Build history of the part. All positions in model axes, mm. A direction names the side the tool comes from. Round coordinates to 2 decimals unless told otherwise and drop trailing zeros. Write each loop counter-clockwise with the first axis right and the second up, starting at its lowest first coordinate (ties: lowest second). Pieces come first, ordered by that corner, then holes. Notation, with made-up numbers: (9, 54.25) -> (47, 54.25) arc R13 cw to (47, 69.25) -> close; hole circle Ø7 at (78.5, 38.5). An arc over 180 degrees is marked (long way). Return JSON: item names as keys, results as strings.
from build123d import *

# Parameters (mm, degrees)
ESQUISSE1_R       = 12
EXTRUSION1_DEPTH  = 12
ESQUISSE2_R       = 15.5
EXTRUSION2_DEPTH  = 2.5
ESQUISSE3_R       = 9
EXTRUSION3_DEPTH  = 1
D_ME1_FACE_RADIUS = 9
D_ME1_HEIGHT      = 6


with BuildPart() as part:
    # Esquisse1 → Extrusion1 (new body)
    with BuildSketch(Plane.XY):
        Circle(ESQUISSE1_R)
    extrude(amount=EXTRUSION1_DEPTH)

    # Esquisse2 → Extrusion2 (add)
    with BuildSketch(Plane.XY.offset(12)):
        Circle(ESQUISSE2_R)
    extrude(amount=EXTRUSION2_DEPTH)

    # Esquisse3 → Extrusion3 (add)
    with BuildSketch(Plane.XY.offset(14.5)):
        Circle(ESQUISSE3_R)
    extrude(amount=EXTRUSION3_DEPTH)

    # Dôme1: a dome of height H over a round flat face of radius A is a cap of a sphere of radius (A * A + H * H) / (2 * H)
    d_me1_r = (D_ME1_FACE_RADIUS * D_ME1_FACE_RADIUS + D_ME1_HEIGHT * D_ME1_HEIGHT) / (2 * D_ME1_HEIGHT)
    d_me1_base = Plane((0, 0, 15.5), z_dir=(0, 0, 1))
    with Locations(d_me1_base.offset(D_ME1_HEIGHT - d_me1_r)):
        d_me1_ball = Sphere(d_me1_r, mode=Mode.PRIVATE)
    add(split(d_me1_ball, bisect_by=d_me1_base, keep=Keep.TOP, mode=Mode.PRIVATE))


solid = part.part
Q1. Saw through at D-D on y = 11. List the corners of the cut face in (x, z).
Verdict:
{"outline": "(-10.92, 12) -> (-4.8, 12) -> (-4.8, 0) -> (4.8, 0) -> (4.8, 12) -> (10.92, 12) -> (10.92, 14.5) -> (-10.92, 14.5) -> close"}
Q2. Wall check: L1, parallel to Z at x = 14.5, y = 0; L2, parallel to Z at x = 8, y = -7; L3, parallel to X at y = -5, z = 9.5. Give the ranges that are in metal, low to high.
Verdict:
{"L1": "z = 12 to 14.5", "L2": "z = 0 to 14.5", "L3": "x = -10.91 to 10.91"}
Q3. Saw through at C-C on z = 11.5. List the corners of the cut face in (x, y), then the cut area to 3 significant figures.
Verdict:
{"outline": "circle Ø24 at (0, 0)", "area": "452 mm²"}
Q4. Saw through at A-A on x = 0. List the corners of the cut face in (y, z), then the cut area to 3 significant figures.
Verdict:
{"outline": "(-15.5, 12) -> (-12, 12) -> (-12, 0) -> (12, 0) -> (12, 12) -> (15.5, 12) -> (15.5, 14.5) -> (9, 14.5) -> (9, 15.5) arc R9.75 ccw to (-9, 15.5) -> (-9, 14.5) -> (-15.5, 14.5) -> close", "area": "462 mm²"}
Q5. Pin check, flat tips, straight feed: pin 1 Ø6 at (y, z) = (4, 11.5) entering from -X; pin 2 Ø10 at (x, z) = (0, 6) entering from +Y; pin 3 Ø3 at (x, z) = (4.5, 4) entering from -Y. Stop position of each tip, or through.
Verdict:
{"pin 1": "stops at x = -15.46", "pin 2": "stops at y = 12", "pin 3": "stops at y = -11.62"}
Q6. 3-axis set-ups, long thin cutter, end or side, ignore diameter. For faces 1 (the cylindrical face through (-11.99, 0.53, 5.92)), 2 (the cylindrical face through (-2.018, 15.368, 13.232)), 3 (the cylindrical face through (-1.172, 8.923, 14.993)): which of +Z, -Z, +X, -X, +Y, -Y reach the whole face in a straight line?
Verdict:
{"face 1": "-Z", "face 2": "+Z, -Z", "face 3": "+Z"}
